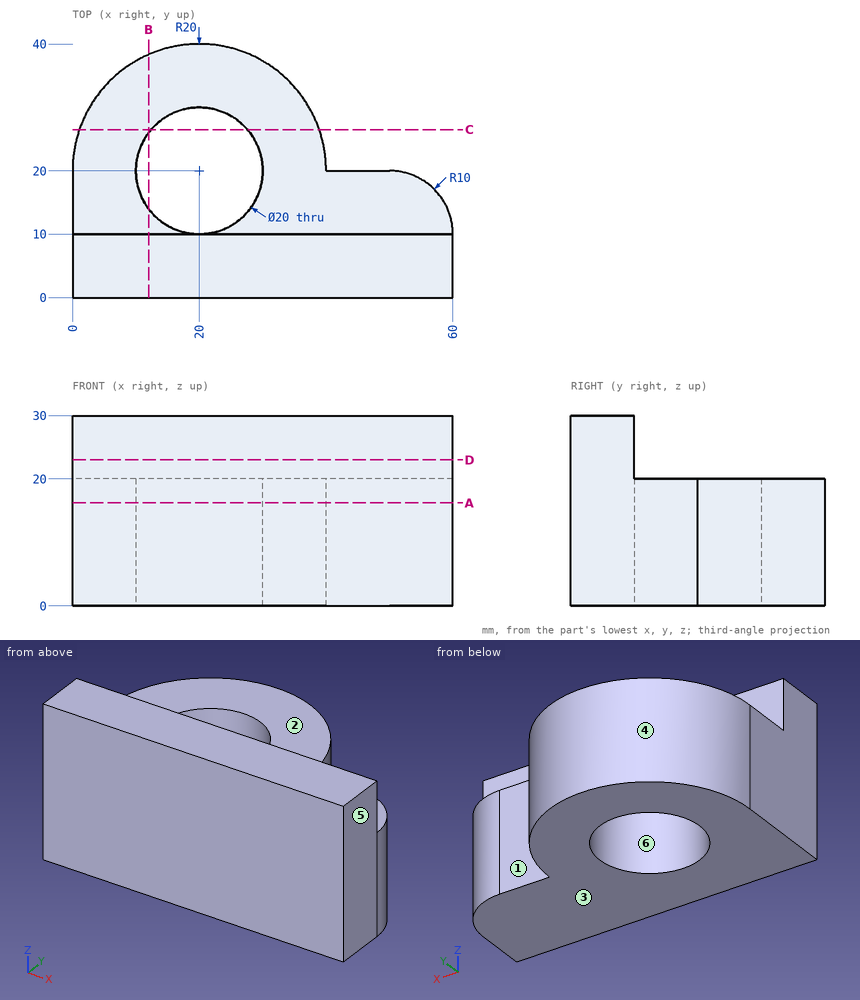
Here's the drawing with two shaded views (mm, measured from the low corner). I have some questions. A direction names the side the tool comes from. Round coordinates to 2 decimals unless told otherwise and drop trailing zeros. Loops run counter-clockwise (first coordinate to the right, second up) from the corner with the lowest first, then second, coordinate; pieces in that order, holes last.
Item 1: Suppose I cut it at B-B, the plane x = 12. Write out the boundary of the cut face in (y, z).
Item 2: Suppose I cut it at D-D, the plane z = 23. Write out the boundary of the cut face in (x, y).
Item 3: Which directions (+Z, -Z, +X, -X, +Y, -Y) give clear straight access to the entire face, cutting with the end or side of a thin tool? Please do the marked faces 1, 2 and 3.
Item 4: Suppose I cut it at C-C, the plane y = 26.5. Write out the boundary of the cut face in (x, z), then the cut area to 3 significant figures.
Item 5: If we mould it in two halves opening along Y, with no side actions, what happens to the marked faces 4, 5 and 6? For each: +Y half, -Y half, draft (parallel to the pull), parting line (faces both ways), or undercut.
Item 6: Will these pins go through, and if not, where does the flat tip stop? pin 1 Ø15 at (x, y) = (34, 26.5) entering from +Z; pin 2 Ø5 at (x, z) = (30, 14.5) entering from +Y; pin 3 Ø11 at (x, z) = (44, 6) entering from +Y; pin 4 Ø8 at (x, y) = (16, 20) entering from -Z.
Item 7: Suppose I cut it at A-A, the plane z = 16.25. Write out the boundary of the cut face in (x, y).
Item 8: Please list where these lines run through material, in increasing order: L1, parallel to Y at x = 20, z = 4.75; L2, parallel to Y at x = 28.5, z = 13; L3, parallel to Z at x = 29, y = 37.
Reported:
1. outline: (0, 0) - (14, 0) - (14, 20) - (10, 20) - (10, 30) - (0, 30) - close; (26, 0) - (38.33, 0) - (38.33, 20) - (26, 20) - close
2. outline: (0, 0) - (60, 0) - (60, 10) - (0, 10) - close
3. face 1: +Z, -Z, +X, +Y
3. face 2: +Z, +X, -X, +Y
3. face 3: -Z, +X, -X, +Y, -Y
4. outline: (1.09, 0) - (12.4, 0) - (12.4, 20) - (1.09, 20) - close; (27.6, 0) - (38.91, 0) - (38.91, 20) - (27.6, 20) - close
4. area: 453 mm2
5. face 4: +Y half
5. face 5: draft
5. face 6: undercut
6. pin 1: stops at z = 20
6. pin 2: stops at y = 38.54
6. pin 3: stops at y = 27.6
6. pin 4: passes through
7. outline: (0, 0) - (60, 0) - (60, 10) arc R10 ccw to (50, 20) - (40, 20) arc R20 ccw to (0, 20) - close; hole circle Ø20 at (20, 20)
8. L1: y = 0 to 10, 30 to 40
8. L2: y = 0 to 14.73, 25.27 to 38.1
8. L3: z = 0 to 20
